Design review of the part built by this model. Coordinates are the model's own, in mm. Face numbers are marked on the shaded views. A direction names the side the tool comes from. Round coordinates to 2 decimals unless told otherwise and drop trailing zeros. Loops run counter-clockwise (first coordinate to the right, second up) from the corner with the lowest first, then second, coordinate; pieces in that order, holes last. Notation, with made-up numbers: (-7.5, -8.75) - (29.5, -8.75) arc R24 cw to (29.5, 10.25) - close; hole circle Ø8 at (-23.5, -10). An arc over 180 degrees is marked (long way). Return JSON: item names as keys, results as strings. Group by question number.
from build123d import *

# Parameters (mm, degrees)
F0_W     = 127
F0_H     = 203.2
F1_DEPTH = 127
F3_DEPTH = 203.2
F4_R     = 15.875
F5_DEPTH = 25.4


with BuildPart() as f1:
    # F0 (on Front) → F1 (new body)
    with BuildSketch(Plane.XZ):
        with Locations((-4.624575, 31.5007)):
            Rectangle(F0_W, F0_H)
    extrude(amount=F1_DEPTH)

    # F2 (on face) → F3 (cut)
    with BuildSketch(Plane.XY.offset(133.1007)):
        Polygon((-49.074575, -107.95), (39.825425, -107.95), (39.825425, -19.05), (27.125425, -19.05), (27.125425, 0), (-36.374575, 0), (-36.374575, -19.05), (-49.074575, -19.05), align=None)
    extrude(amount=-F3_DEPTH, mode=Mode.SUBTRACT)

    # F4 (on face) → F5 (cut)
    with BuildSketch(Plane.XZ.offset(127)):
        with Locations((0, 104.891345)):
            Circle(F4_R)
    extrude(amount=-F5_DEPTH, mode=Mode.SUBTRACT)


solid = f1.part
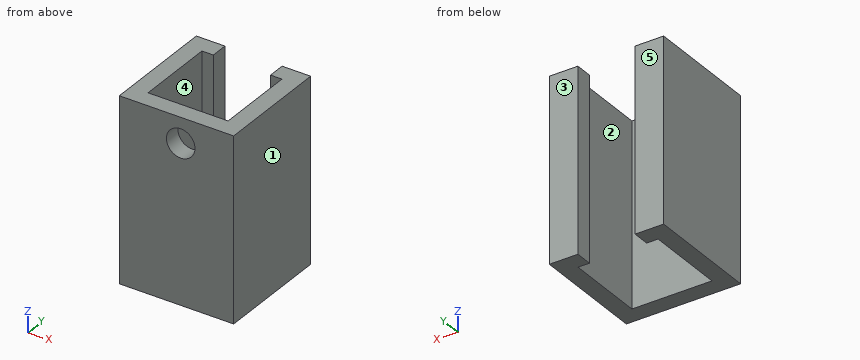
Q1. Tool access review of the marked faces 4 and 5: name each direction out of +Z, -Z, +X, -X, +Y, -Y from which nothing blocks a thin tool from reaching the whole face with its end or side.
Q2. Add section B-B, the plane x = 0. State the section outline as (y, z) points, plus the area to 3 significant figures.
Q3. For line 1 (X direction, y = -21, z = 46); line 2 (Y direction, x = 29, z = 69.5); line 3 (X direction, y = -9.5, z = -9.5), list the stretches that pass through material, from the lowest coordinate up.
Q4. Insertion check: pin 1 Ø12 at (x, y) = (30.5, -88.5) entering from -Z; pin 2 Ø10 at (x, z) = (-29, -37.5) entering from +Y. Each pin has a flat end and moves straight along its axis. Give the tip position at first contact, or say it passes through.
Q5. Add section D-D, the plane z = -52. State the section outline as (x, y) points.
Q6. Add section A-A, the plane y = -16.5. State the section outline as (x, z) points, plus the area to 3 significant figures.
Q7. Draft analysis for pull direction Y (two halves, no side actions). For the marked faces 1, 2 and 3, state which applies: pulls with the +Y half, pulls with the -Y half, needs draft (parallel to the pull), parting line crosses it, or undercut.
Q8. Add section C-C, the plane z = 108.5. State the section outline as (x, y) points, plus the area to 3 significant figures.
Evaluation:
{
 "1": {"face 4": "+Z, -Z", "face 5": "+Z, -Z, +X, -X, +Y"},
 "2": {"outline": "(-127, -70.1) - (-107.95, -70.1) - (-107.95, 89.02) - (-127, 89.02) - close; (-127, 120.77) - (-107.95, 120.77) - (-107.95, 133.1) - (-127, 133.1) - close", "area": "3,270 mm²"},
 "3": {"line 1": "-68.12 to -49.07, 39.83 to 58.88", "line 2": "-127 to -107.95, -19.05 to 0", "line 3": "-68.12 to -36.37, 27.13 to 58.88"},
 "4": {"pin 1": "through", "pin 2": "y = -107.95"},
 "5": {"outline": "(-68.12, -127) - (58.88, -127) - (58.88, 0) - (27.13, 0) - (27.13, -19.05) - (39.83, -19.05) - (39.83, -107.95) - (-49.07, -107.95) - (-49.07, -19.05) - (-36.37, -19.05) - (-36.37, 0) - (-68.12, 0) - close"},
 "6": {"outline": "(-68.12, -70.1) - (-36.37, -70.1) - (-36.37, 133.1) - (-68.12, 133.1) - close; (27.13, -70.1) - (58.88, -70.1) - (58.88, 133.1) - (27.13, 133.1) - close", "area": "12,900 mm²"},
 "7": {"face 1": "needs draft", "face 2": "undercut", "face 3": "pulls with the +Y half"},
 "8": {"outline": "(-68.12, -127) - (-15.46, -127) - (-15.46, -107.95) - (-49.07, -107.95) - (-49.07, -19.05) - (-36.37, -19.05) - (-36.37, 0) - (-68.12, 0) - close; (15.46, -127) - (58.88, -127) - (58.88, 0) - (27.13, 0) - (27.13, -19.05) - (39.83, -19.05) - (39.83, -107.95) - (15.46, -107.95) - close", "area": "6,430 mm²"}
}
